Read the model definition and answer for the solid it produces. Units are mm, in the model's axes. A direction names the side the tool comes from. Give positions to 0.01 mm unless a question says otherwise; leave off trailing zeros. Write each loop counter-clockwise with the first axis right and the second up, starting at its lowest first coordinate (ties: lowest second). Pieces come first, ordered by that corner, then holes.
```python
from build123d import *

# Parameters (mm, degrees)
CROQUIS1_R              = 18.4
SALIENTE_EXTRUIR1_DEPTH = 26.3
CROQUIS2_R              = 3
CROQUIS2_R_2            = 1.25
CORTAR_EXTRUIR1_DEPTH   = 5
CROQUIS3_R              = 1.25
CORTAR_EXTRUIR2_DEPTH   = 5


with BuildPart() as part:
    # Croquis1 → Saliente-Extruir1 (new body)
    with BuildSketch(Plane.XY):
        Circle(CROQUIS1_R)
    extrude(amount=SALIENTE_EXTRUIR1_DEPTH)

    # Croquis2 → Cortar-Extruir1 (cut)
    with BuildSketch(Plane.XY.offset(26.3)):
        Circle(CROQUIS2_R)
        with Locations((0, 9.5)):
            Circle(CROQUIS2_R_2)
        with Locations((9.5, 0)):
            Circle(CROQUIS2_R_2)
        with Locations((0, -9.5)):
            Circle(CROQUIS2_R_2)
        with Locations((-9.5, 0)):
            Circle(CROQUIS2_R_2)
    extrude(amount=-CORTAR_EXTRUIR1_DEPTH, mode=Mode.SUBTRACT)

    # Croquis3 → Cortar-Extruir2 (cut)
    with BuildSketch(Plane(origin=(0, 0, 0), x_dir=(-1, 0, 0), z_dir=(0, 0, -1))):
        with Locations((-10, 0)):
            Circle(CROQUIS3_R)
        with Locations((0, 10)):
            Circle(CROQUIS3_R)
        with Locations((10, 0)):
            Circle(CROQUIS3_R)
        with Locations((0, -10)):
            Circle(CROQUIS3_R)
    extrude(amount=-CORTAR_EXTRUIR2_DEPTH, mode=Mode.SUBTRACT)


solid = part.part
```
Item 1: Section C-C (z = 19) is taken. Write down the section's boundary in (x, y).
Result set:
outline: circle Ø36.8 at (0, 0)
Item 2: Section A-A (y = 0) is taken. Write down the section's boundary in (x, z), and give its area (3 significant figures).
Result set:
outline: (-18.4, 0) - (-11.25, 0) - (-11.25, 5) - (-8.75, 5) - (-8.75, 0) - (8.75, 0) - (8.75, 5) - (11.25, 5) - (11.25, 0) - (18.4, 0) - (18.4, 26.3) - (10.75, 26.3) - (10.75, 21.3) - (8.25, 21.3) - (8.25, 26.3) - (3, 26.3) - (3, 21.3) - (-3, 21.3) - (-3, 26.3) - (-8.25, 26.3) - (-8.25, 21.3) - (-10.75, 21.3) - (-10.75, 26.3) - (-18.4, 26.3) - close
area: 888 mm2
Item 3: Each of these flat-tipped pins is pushed along its axis until it touches: pin 1 Ø1 at (y, z) = (-12.5, 8.5) entering from +X; pin 2 Ø4 at (x, z) = (1.5, 18) entering from +Y; pin 3 Ø2 at (x, y) = (0, -9.5) entering from +Z. Where does it stop, or does it pass through?
Result set:
pin 1: stops at x = 13.95
pin 2: stops at y = 18.4
pin 3: stops at z = 21.3
Item 4: Determine the mould class of faces 1 (the flat face through (10, 0, 5)), 2 (the flat face through (9, 0, 21.3)), 3 (the flat face through (0, 0, 0)), 4 (the cylindrical face through (-14.6, -11.2, 13)) for opening direction Y: pulls with the +Y half, pulls with the -Y half, needs draft (parallel to the pull), parting line crosses it, or undercut.
Result set:
face 1: undercut
face 2: undercut
face 3: needs draft
face 4: parting line crosses it
Item 5: Section D-D (x = 10) is taken. Write down the section's boundary in (y, z).
Result set:
outline: (-15.45, 0) - (-1.25, 0) - (-1.25, 5) - (1.25, 5) - (1.25, 0) - (15.45, 0) - (15.45, 26.3) - (1.15, 26.3) - (1.15, 21.3) - (-1.15, 21.3) - (-1.15, 26.3) - (-15.45, 26.3) - close
Item 6: Which of the six approach directions +Z, -Z, +X, -X, +Y, -Y give full straight-line access (tool end or side, diameter ignored) to faces 5 (the cylindrical face through (-0.16, 10.74, 23.84)), 6 (the cylindrical face through (0.16, 11.24, 2.46))?
Result set:
face 5: +Z
face 6: -Z
Item 7: Find the intervals of material crossed by line 1 along Y through (x, z) = (0, 22.6); line 2 along Y through (x, z) = (0, 1.35); line 3 along Y through (x, z) = (-10, 3.65), in increasing order.
Result set:
line 1: y = -18.4 to -10.75, -8.25 to -3, 3 to 8.25, 10.75 to 18.4
line 2: y = -18.4 to -11.25, -8.75 to 8.75, 11.25 to 18.4
line 3: y = -15.45 to -1.25, 1.25 to 15.45
